Part print with two shaded views. Sizes in mm from the minimum x, y, z corner. A direction names the side the tool comes from. Coordinates: 2 decimals unless noted, no trailing zeros. Loops run counter-clockwise (first coordinate to the right, second up) from the corner with the lowest first, then second, coordinate; pieces in that order, holes last. Notation, with made-up numbers: (-19, 60) - (25, 60) arc R23 cw to (25, 69) - close; hole circle Ø6 at (-7.75, -2). An arc over 180 degrees is marked (long way). Answer as CSV lines item,"result".
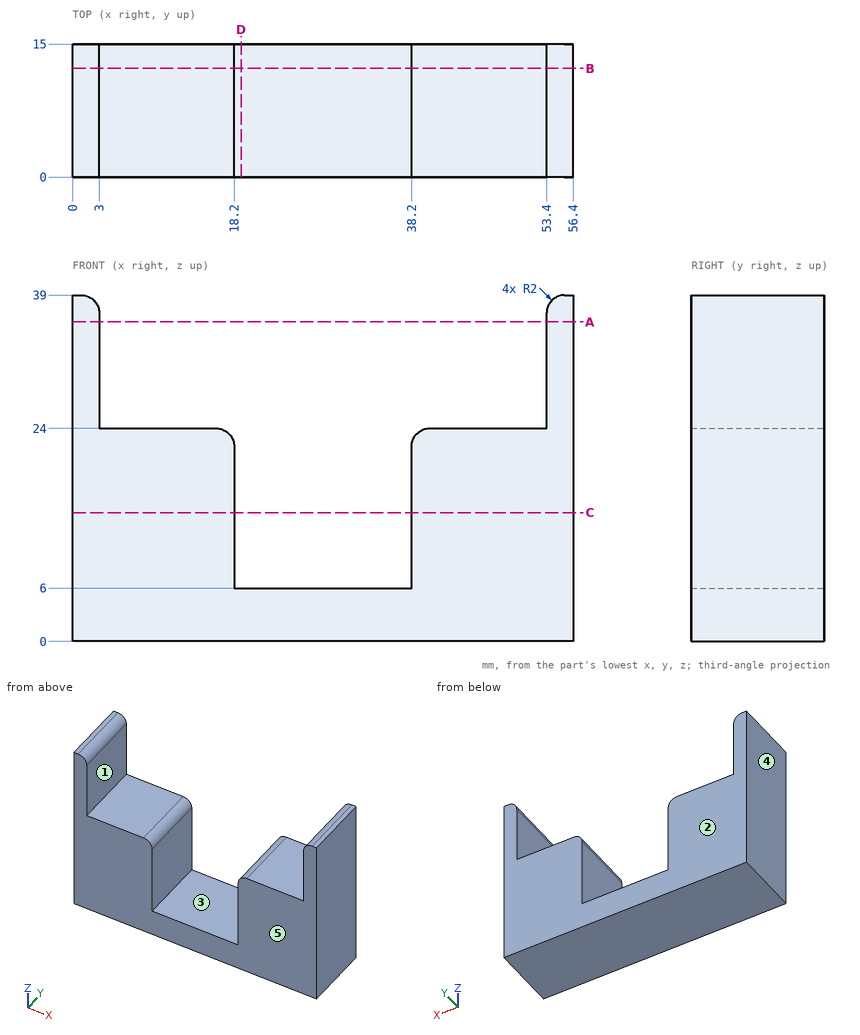
Q1. Saw through at B-B (y = 12.25). Give the cut face in (x, z).
Results:
outline,"(0, 0) - (56.4, 0) - (56.4, 39) - (55.4, 39) arc R2 ccw to (53.4, 37) - (53.4, 24) - (40.2, 24) arc R2 ccw to (38.2, 22) - (38.2, 6) - (18.2, 6) - (18.2, 22) arc R2 ccw to (16.2, 24) - (3, 24) - (3, 37) arc R2 ccw to (1, 39) - (0, 39) - close"
Q2. Two-plate mould, pull along X, no slides. Class the marked faces 3, 4 and 5: released by +X, released by -X, zero draft, split by the parting line, or undercut.
Results:
face 3,"undercut"
face 4,"released by -X"
face 5,"zero draft"
Q3. Saw through at C-C (z = 14.5). Give the cut face in (x, y).
Results:
outline,"(0, 0) - (18.2, 0) - (18.2, 15) - (0, 15) - close; (38.2, 0) - (56.4, 0) - (56.4, 15) - (38.2, 15) - close"
Q4. Which spindle directions (+Z, -Z, +X, -X, +Y, -Y) get a long thin tool onto all of the face, cutting with end or side? Do the marked faces 1 and 2. Say none if no direction does.
Results:
face 1,"+Z, +Y, -Y"
face 2,"+Z, -Z, +X, -X, +Y"
Q5. Flat gauge pins, fed straight in: pin 1 (7.5 mm diameter, centred on x = 25.5, y = 9, fed in from +Z); pin 2 (2 mm diameter, centred on y = 3.5, z = 21.5, fed in from -X); pin 3 (4 mm diameter, centred on x = 47.5, y = 9.5, fed in from +Z). Where does each tip first touch, or does it go through?
Results:
pin 1,"stops at z = 6"
pin 2,"stops at x = 0"
pin 3,"stops at z = 24"
Q6. Saw through at A-A (z = 36). Give the cut face in (x, y).
Results:
outline,"(0, 0) - (3, 0) - (3, 15) - (0, 15) - close; (53.4, 0) - (56.4, 0) - (56.4, 15) - (53.4, 15) - close"
Q7. Wall check: L1, parallel to X at y = 12, z = 33; L2, parallel to X at y = 7, z = 18.5; L3, parallel to Z at x = 7, y = 3. Give the ranges that are in metal, low to high.
Results:
L1,"x = 0 to 3, 53.4 to 56.4"
L2,"x = 0 to 18.2, 38.2 to 56.4"
L3,"z = 0 to 24"
Q8. Saw through at D-D (x = 19). Give the cut face in (y, z).
Results:
outline,"(0, 0) - (15, 0) - (15, 6) - (0, 6) - close"
